Check sheet for the modelled part. Datum: model origin and axes. Units: mm. A direction names the side the tool comes from. Coordinates: 2 decimals unless noted, no trailing zeros. Order: outer loops, then holes, each group sorted by start corner. A loop starts at its lowest first (then second) coordinate and runs counter-clockwise, first axis right, second up.
from build123d import *

# Parameters (mm, degrees)
F0_R     = 5
F0_W     = 5
F0_H     = 15
F0_W_2   = 40
F0_H_2   = 8
F1_DEPTH = 5


# Not quite as in the source:
# - a feature names something its author has since deleted; it is built from what else it names


with BuildPart() as f1:
    # F0 (on Front) → F1 (new body)
    with BuildSketch(Plane.XZ):
        with BuildLine():
            Line((0, 122), (0, 0))
            Line((0, 0), (40, 0))
            Line((40, 0), (42, 0))
            Line((42, 0), (158, 0))
            Line((158, 0), (160, 0))
            Line((160, 0), (200, 0))
            Line((200, 0), (200, 39.7))
            Line((200, 39.7), (159.7, 39.7))
            Line((159.7, 39.7), (143.1136062057, 39.7))
            ThreePointArc((143.1136062057, 39.7), (138.9711431703, 37.5), (134.8286801349, 39.7))
            Line((134.8286801349, 39.7), (100, 39.7))
            ThreePointArc((100, 39.7), (78.0895572843, 52.35), (78.0895572843, 77.65))
            ThreePointArc((78.0895572843, 77.65), (87.35, 86.9104427157), (100, 90.3))
            Line((100, 90.3), (159.7, 90.3))
            Line((159.7, 90.3), (200, 90.3))
            Line((200, 90.3), (200, 122))
            Line((200, 122), (160, 122))
            Line((160, 122), (158, 130))
            Line((158, 130), (42, 130))
            Line((42, 130), (40, 122))
            Line((40, 122), (0, 122))
        make_face()
        with Locations((20, 20)):
            Circle(F0_R, mode=Mode.SUBTRACT)
        with Locations((31.5, 28.75)):
            Rectangle(F0_W, F0_H, mode=Mode.SUBTRACT)
        with Locations((180, 20)):
            Circle(F0_R, mode=Mode.SUBTRACT)
        with Locations((31.5, 65)):
            Rectangle(F0_W, F0_H, mode=Mode.SUBTRACT)
        with BuildLine():
            ThreePointArc((66.0288568297, 87.5), (65.8584859611, 86.2059047745), (65.3589838486, 85))
            ThreePointArc((65.3589838486, 85), (56.1992276983, 88.7940952255), (66.0288568297, 87.5))
        make_face(mode=Mode.SUBTRACT)
        with Locations((20, 110)):
            Circle(F0_R, mode=Mode.SUBTRACT)
        with Locations((31.5, 101.25)):
            Rectangle(F0_W, F0_H, mode=Mode.SUBTRACT)
        with Locations((180, 110)):
            Circle(F0_R, mode=Mode.SUBTRACT)
        with BuildLine():
            ThreePointArc((66.0288568297, 87.5), (56.1992276983, 88.7940952255), (65.3589838486, 85))
            ThreePointArc((65.3589838486, 85), (65.8584859611, 86.2059047745), (66.0288568297, 87.5))
        make_face()
        with Locations((20, 126)):
            Rectangle(F0_W_2, F0_H_2)
        with Locations((180, 126)):
            Rectangle(F0_W_2, F0_H_2)
        Polygon((160, 130), (158, 130), (160, 122), align=None)
        Polygon((40, 130), (40, 122), (42, 130), align=None)
        with BuildLine():
            ThreePointArc((134.8286801349, 39.7), (138.9711431703, 37.5), (143.1136062057, 39.7))
            Line((143.1136062057, 39.7), (134.8286801349, 39.7))
        make_face()
    extrude(amount=F1_DEPTH)


solid = f1.part
(1) Release check for a two-part mould opening along X. For faces 4 (the cylindrical face through (18.92, -2.46, 105.12)), 5 (the flat face through (101, -2, 130)), 6 (the flat face through (200, -2, 110)) record: +X half, -X half, draft (parallel to the pull), parting line (faces both ways), or undercut.
Filled in:
face 4: undercut
face 5: draft
face 6: +X half
(2) Thickness scan on probe 1 along X at (y, z) = (-2.85, 20.5); probe 2 along Z at (x, y) = (20, -2.6); probe 3 along Z at (x, y) = (180, -2.2). Record the ranges inside material, lowest first.
Filled in:
probe 1: x = 0 to 15.03, 24.97 to 175.03, 184.97 to 200
probe 2: z = 0 to 15, 25 to 105, 115 to 130
probe 3: z = 0 to 15, 25 to 39.7, 90.3 to 105, 115 to 130
(3) Cross-section at A-A (x = 124.5). Enter the section's corners in (y, z), and give its area (3 significant figures).
Filled in:
outline: (-5, 0) - (0, 0) - (0, 39.7) - (-5, 39.7) - close; (-5, 90.3) - (0, 90.3) - (0, 130) - (-5, 130) - close
area: 397 mm2
(4) Cross-section at C-C (x = 180). Enter the section's corners in (y, z).
Filled in:
outline: (-5, 0) - (0, 0) - (0, 15) - (-5, 15) - close; (-5, 25) - (0, 25) - (0, 39.7) - (-5, 39.7) - close; (-5, 90.3) - (0, 90.3) - (0, 105) - (-5, 105) - close; (-5, 115) - (0, 115) - (0, 130) - (-5, 130) - close
(5) Cross-section at B-B (y = -0.9). Enter the section's corners in (x, z).
Filled in:
outline: (0, 0) - (200, 0) - (200, 39.7) - (100, 39.7) arc R25.3 cw to (100, 90.3) - (200, 90.3) - (200, 130) - (0, 130) - close; hole circle Ø10 at (20, 20); hole circle Ø10 at (20, 110); hole (29, 21.25) - (34, 21.25) - (34, 36.25) - (29, 36.25) - close; hole (29, 57.5) - (34, 57.5) - (34, 72.5) - (29, 72.5) - close; hole (29, 93.75) - (34, 93.75) - (34, 108.75) - (29, 108.75) - close; hole circle Ø10 at (180, 20); hole circle Ø10 at (180, 110)
(6) Go/stop test with a flat-tipped pin: P1, Ø1.5, axis at y = -1, z = 44, coming from the +X side. Record where the tip stops, or that it passes through.
Filled in:
P1: stops at x = 87.08
(7) Tool access check on faces 1 (the flat face through (0, -2, 66)), 2 (the flat face through (31, -2, 57.5)), 3 (the flat face through (149, -2, 90.3)). Record the directions out of +Z, -Z, +X, -X, +Y, -Y that give a thin tool (end or side, any length) a straight path to the whole face; none if there is none.
Filled in:
face 1: +Z, -Z, -X, +Y, -Y
face 2: +Y, -Y
face 3: +X, +Y, -Y
(8) Cross-section at D-D (x = 20). Enter the section's corners in (y, z), and give its area (3 significant figures).
Filled in:
outline: (-5, 0) - (0, 0) - (0, 15) - (-5, 15) - close; (-5, 25) - (0, 25) - (0, 105) - (-5, 105) - close; (-5, 115) - (0, 115) - (0, 130) - (-5, 130) - close
area: 550 mm2
